Here's how the part is built. I have some questions about the finished solid (model axes, mm). Round coordinates to 2 decimals unless told otherwise and drop trailing zeros. Write each loop counter-clockwise with the first axis right and the second up, starting at its lowest first coordinate (ties: lowest second). Pieces come first, ordered by that corner, then holes. Notation, with made-up numbers: (15.5, 51) -> (64.5, 51) arc R35 cw to (64.5, 85) -> close; hole circle Ø4 at (81.5, 24). An arc over 180 degrees is marked (long way). Put each result on its own line as item: value. Start each with the question number.
1) I want a section at A-A, the plane y = 25. List the corners of the cut face in (x, z) for me, then the cut area to 3 significant figures.
2) If I drill on line 1 along Y through (x, z) = (251, 10.75); line 2 along X through (y, z) = (371.5, 16); line 3 along Y through (x, z) = (220, 19.75), over which ranges is the centre line in solid material (lowest first)? Write a range as [from, to].
3) Will these pins go through, and if not, where does the flat tip stop? P1, Ø3, axis at y = 112, z = 2.5, coming from the -X side; P2, Ø7.5, axis at x = 251, y = 375, coming from the -Z side; P3, Ø12, axis at x = 54.405, y = 125, coming from the +Z side; P4, Ø4, axis at x = 117, z = 3, coming from the -Y side.
4) I want a section at B-B, the plane x = 17. List the corners of the cut face in (y, z) for me.
from build123d import *

# Parameters (mm, degrees)
CROQUIS1_W                         = 268
CROQUIS1_H                         = 400
CROQUIS1_R                         = 4
SALIENTE_EXTRUIR1_DEPTH            = 25
CROQUIS2_R                         = 10
CORTAR_EXTRUIR1_DEPTH              = 7
REDONDEO1_R                        = 10
REDONDEO2_R                        = 10
CROQUIS3_R                         = 10
CORTAR_EXTRUIR2_DEPTH              = 7
TALADRO_DE_MARGEN_PARA_5_161_D     = 8.4328
TALADRO_DE_MARGEN_PARA_5_161_DEPTH = 18


with BuildPart() as part:
    # Croquis1 → Saliente-Extruir1 (new body)
    with BuildSketch(Plane.XY):
        with Locations((134, 200)):
            Rectangle(CROQUIS1_W, CROQUIS1_H)
        with Locations((54.405, 275)):
            Circle(CROQUIS1_R, mode=Mode.SUBTRACT)
        with Locations((213.605, 275)):
            Circle(CROQUIS1_R, mode=Mode.SUBTRACT)
        with Locations((213.605, 125)):
            Circle(CROQUIS1_R, mode=Mode.SUBTRACT)
        with Locations((54.405, 125)):
            Circle(CROQUIS1_R, mode=Mode.SUBTRACT)
    extrude(amount=SALIENTE_EXTRUIR1_DEPTH)

    # Croquis2 → Cortar-Extruir1 (cut)
    with BuildSketch(Plane.XY.offset(25)):
        with Locations((54.405, 275)):
            Circle(CROQUIS2_R)
        with Locations((213.605, 275)):
            Circle(CROQUIS2_R)
        with Locations((213.605, 125)):
            Circle(CROQUIS2_R)
        with Locations((54.405, 125)):
            Circle(CROQUIS2_R)
    extrude(amount=-CORTAR_EXTRUIR1_DEPTH, mode=Mode.SUBTRACT)

    # Redondeo1
    redondeo1_edges = [part.edges().sort_by_distance(p)[0] for p in [
        (0, 400, 12.5),
        (268, 400, 12.5),
        (268, 0, 12.5),
        (0, 0, 12.5),
    ]]
    fillet(redondeo1_edges, radius=REDONDEO1_R)

    # Redondeo2
    redondeo2_edges = [part.edges().sort_by_distance(p)[0] for p in [
        (268, 200, 0),
        (0, 200, 0),
        (134, 400, 0),
        (134, 0, 0),
        (2.928932188, 397.071067812, 0),
        (265.071067812, 397.071067812, 0),
        (2.928932188, 2.928932188, 0),
        (265.071067812, 2.928932188, 0),
    ]]
    fillet(redondeo2_edges, radius=REDONDEO2_R)

    # Croquis3 → Cortar-Extruir2 (cut)
    with BuildSketch(Plane.XY.offset(25)):
        with Locations((17, 375)):
            Circle(CROQUIS3_R)
        with Locations((251, 375)):
            Circle(CROQUIS3_R)
        with Locations((251, 25)):
            Circle(CROQUIS3_R)
        with Locations((17, 25)):
            Circle(CROQUIS3_R)
    extrude(amount=-CORTAR_EXTRUIR2_DEPTH, mode=Mode.SUBTRACT)

    # Taladro de margen para 5/161
    with Locations(Plane.XY.offset(18)):
        with Locations((17, 25), (251, 25), (251, 375), (17, 375)):
            Hole(TALADRO_DE_MARGEN_PARA_5_161_D / 2, depth=TALADRO_DE_MARGEN_PARA_5_161_DEPTH)


solid = part.part
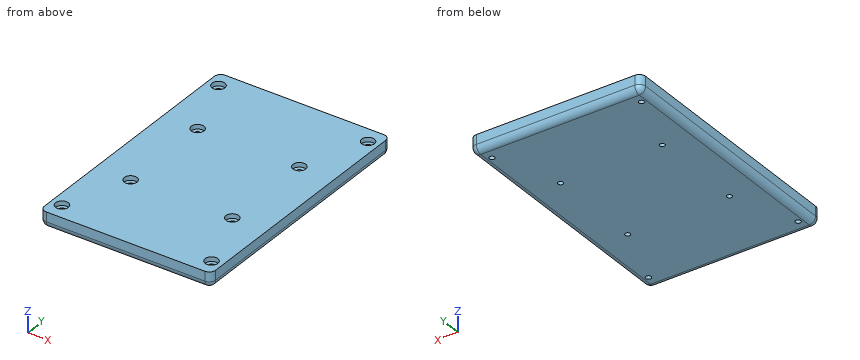
Findings:
1. outline: (0, 10) arc R10 ccw to (10, 0) -> (12.78, 0) -> (12.78, 18) -> (7, 18) -> (7, 25) -> (0, 25) -> close; (21.22, 0) -> (246.78, 0) -> (246.78, 18) -> (241, 18) -> (241, 25) -> (27, 25) -> (27, 18) -> (21.22, 18) -> close; (255.22, 0) -> (258, 0) arc R10 ccw to (268, 10) -> (268, 25) -> (261, 25) -> (261, 18) -> (255.22, 18) -> close
1. area: 6,070 mm2
2. line 1: y = [0, 20.78], [29.22, 370.78], [379.22, 400]
2. line 2: x = [0, 14.65], [19.35, 248.65], [253.35, 268]
2. line 3: y = [0, 117.31], [132.69, 267.31], [282.69, 400]
3. P1: stops at x = 2
3. P2: passes through
3. P3: stops at z = 18
3. P4: stops at y = 1.34
4. outline: (0, 10) arc R10 ccw to (10, 0) -> (20.78, 0) -> (20.78, 18) -> (15, 18) -> (15, 25) -> (0, 25) -> close; (29.22, 0) -> (370.78, 0) -> (370.78, 18) -> (365, 18) -> (365, 25) -> (35, 25) -> (35, 18) -> (29.22, 18) -> close; (379.22, 0) -> (390, 0) arc R10 ccw to (400, 10) -> (400, 25) -> (385, 25) -> (385, 18) -> (379.22, 18) -> close
